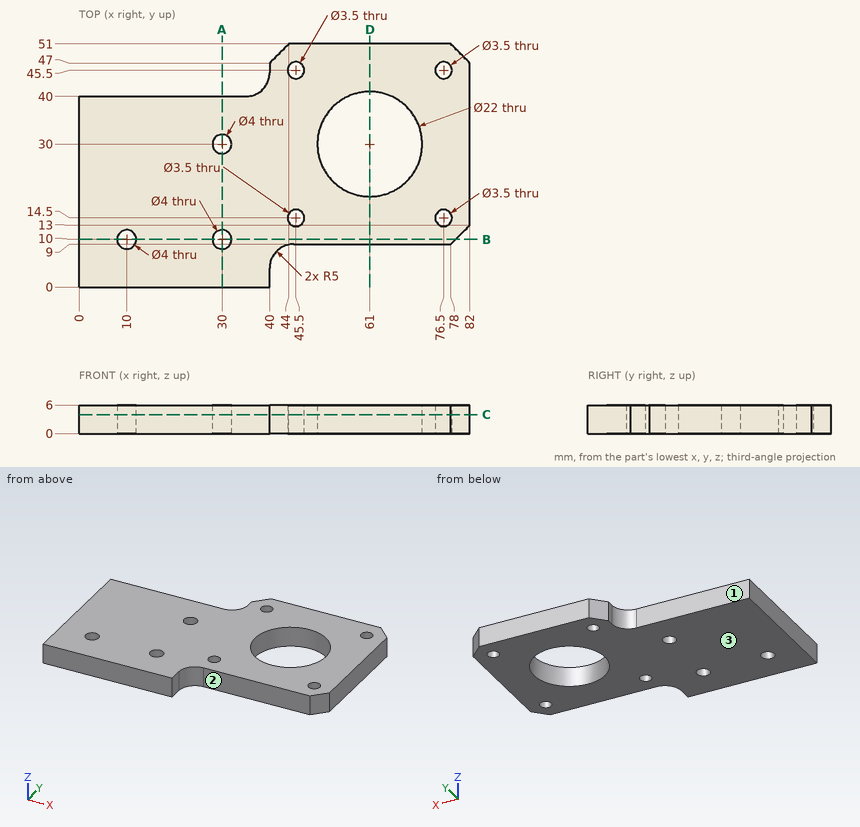
Here's the drawing with two shaded views (mm, measured from the low corner). I have some questions. A direction names the side the tool comes from. Give positions to 0.01 mm unless a question says otherwise; leave off trailing zeros. Write each loop counter-clockwise with the first axis right and the second up, starting at its lowest first coordinate (ties: lowest second). Pieces come first, ordered by that corner, then holes. Notation, with made-up numbers: (67.5, 51) - (105.5, 51) arc R11 cw to (105.5, 59) - close; hole circle Ø6 at (-12, 68.5). An arc over 180 degrees is marked (long way). One line per item, written item: value. Start each with the question number.
Item 1: Imagine slicing it at A-A, the plane x = 30. List the corners of the cut face in (y, z) for me, and give its area (3 significant figures).
Item 2: Imagine slicing it at D-D, the plane x = 61. List the corners of the cut face in (y, z) for me.
Item 3: Imagine slicing it at C-C, the plane z = 4. Give the number of separate pieces and of enclosed holes in the cut face, and give its area (3 significant figures).
Item 4: Imagine slicing it at B-B, the plane y = 10. List the corners of the cut face in (x, z) for me, and give its area (3 significant figures).
Item 5: I'm going to push flat-ended pins straight in: pin 1 (2 mm diameter, centred on y = 46, z = 3.5, fed in from -X); pin 2 (1.8 mm diameter, centred on x = 25.5, z = 3.5, fed in from +Y); pin 3 (3 mm diameter, centred on x = 66.5, z = 2, fed in from -Y). Where does each tip first touch, or does it pass through?
Item 6: Which directions (+Z, -Z, +X, -X, +Y, -Y) give clear straight access to the entire face, cutting with the end or side of a thin tool? Please do the marked faces 1, 2 and 3.
Item 7: Please list where these lines run through material, in increasing order: line 1 (Y direction, x = 30, z = 3.05); line 2 (Y direction, x = 76.5, z = 2.15); line 3 (X direction, y = 46, z = 1). Write a range as from..to.
Geometry says:
1. outline: (0, 0) - (8, 0) - (8, 6) - (0, 6) - close; (12, 0) - (28, 0) - (28, 6) - (12, 6) - close; (32, 0) - (40, 0) - (40, 6) - (32, 6) - close
1. area: 192 mm^2
2. outline: (9, 0) - (19, 0) - (19, 6) - (9, 6) - close; (41, 0) - (51, 0) - (51, 6) - (41, 6) - close
3. separate pieces: 1
3. enclosed holes: 8
3. area: 2,890 mm^2
4. outline: (0, 0) - (8, 0) - (8, 6) - (0, 6) - close; (12, 0) - (28, 0) - (28, 6) - (12, 6) - close; (32, 0) - (79, 0) - (79, 6) - (32, 6) - close
4. area: 426 mm^2
5. pin 1: x = 40
5. pin 2: y = 40
5. pin 3: y = 9
6. face 1: +Z, -Z, -X, +Y
6. face 2: +Z, -Z, +X, -Y
6. face 3: -Z, +X, -X, +Y, -Y
7. line 1: 0..8, 12..28, 32..40
7. line 2: 9..12.75, 16.25..43.75, 47.25..51
7. line 3: 40..43.82, 47.18..74.82, 78.18..82
